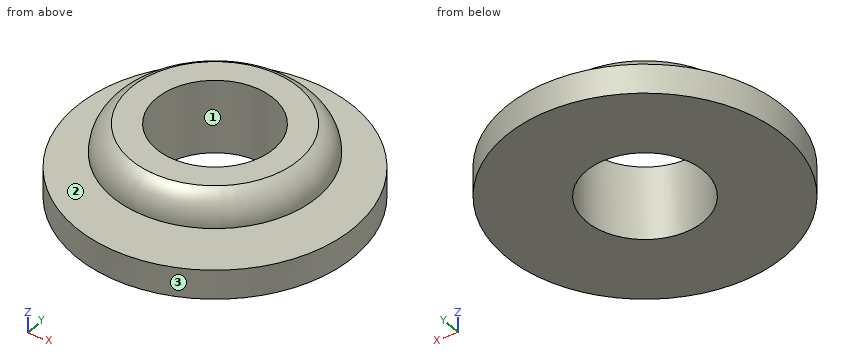
Solid Edge part; units mm, degrees
sketch "Sketch1" plane through (0, 0, 0) normal (0, 0, -1) x (-1, 0, 0)
  circle A0 centre (0, 0) radius 9.5
extrude "Protrusion1" add sketch "Sketch1" along normal blind 5
sketch "Sketch2" plane through (0, 0, -5) normal (0, 0, -1) x (1, 0, 0)
  circle A0 centre (0, 0) radius 4
extrude "Kivágás_1" cut sketch "Sketch2" against normal blind 7.7152
sketch "Sketch3" plane through (0, 0, 0) normal (0, 1, 0) x (-1, 0, 0)
  line L0 (-9.5, -3) -> (-7, -3)
  line L1 (-7, -3) -> (-5, -3)
  line L2 (-5, -3) -> (-5, -2)
  line L3 (-5, -2) -> (-7, -2)
  arc A0 (-7, -2) -> (-5.725, 0) centre (-4.7939, -2) cw
  line L4 (-5.6957, 1.469) -> (-5.725, 0)
  line L5 (-11.4658, 1.2586) -> (-5.6957, 1.469)
  line L6 (-12.1673, -3) -> (-11.4658, 1.2586)
  line L7 (-9.5, -3) -> (-12.1673, -3)
revolve "RevolvedCutout1" cut sketch "Sketch3" angle 360 about axis through (0, 0, 0) along (0, 0, 1)
properties material "Réz, sárgaréz"
Geometry: final body of the model. Coordinates: model frame, mm. Face numbers are marked on the shaded views. Round coordinates to 2 decimals unless told otherwise and drop trailing zeros. Loops run counter-clockwise (first coordinate to the right, second up) from the corner with the lowest first, then second, coordinate; pieces in that order, holes last.
Q1. Section C-C on z = -0.55. Return loops of the section in (x, y).
Q2. Pin query (flat end, axial travel): P1, Ø1.5, axis at x = -2.5, z = -3.5, coming from the -Y side; P2, Ø1, axis at x = 5, y = -6, coming from the +Z side; P3, Ø1, axis at x = 5.5, z = -3, coming from the +Y side. Return the tip coordinate at first contact, or that it passes through.
Q3. Pull-direction query (X, two-part tool) for the marked faces 1, 2 and 3; classes: released by +X, released by -X, zero draft, split by the parting line, or undercut.
Q4. Material intervals for L1, parallel to Y at x = 0, z = -3.85; L2, parallel to Y at x = 0, z = -2.7; L3, parallel to Z at x = -5.25, y = -7.75, sorted ascending.
Q5. Section B-B on y = -7.5. Return loops of the section in (x, z), plus the area to 3 significant figures.
Q6. Section A-A on z = -2.7. Return loops of the section in (x, y).
Evaluation:
1. outline: circle Ø12.91 at (0, 0); hole circle Ø8 at (0, 0)
2. P1: stops at y = -9.34
2. P2: stops at z = -3
2. P3: stops at y = 8.08
3. face 1: undercut
3. face 2: zero draft
3. face 3: split by the parting line
4. L1: y = -9.5 to -4, 4 to 9.5
4. L2: y = -5 to -4, 4 to 5
4. L3: z = -5 to -3
5. outline: (-5.83, -5) - (5.83, -5) - (5.83, -3) - (-5.83, -3) - close
5. area: 23.3 mm2
6. outline: circle Ø10 at (0, 0); hole circle Ø8 at (0, 0)
